Could you check a few things on this model? Use its own coordinates, in mm. A direction names the side the tool comes from. Give positions to 0.01 mm unless a question says otherwise; leave off trailing zeros. Loops run counter-clockwise (first coordinate to the right, second up) from the corner with the lowest first, then second, coordinate; pieces in that order, holes last. Notation, with made-up numbers: M 41.5,-28 L 99.5,-28 A29 cw 99.5,6 Z; hole C 68.25,7 d8. An arc over 180 degrees is marked long. Use a Markdown table: item, result. Add a question column.
1) Will this pin go through, and if not, where does the flat tip stop? pin 1 Ø2 at (x, z) = (3, -3) entering from +Y.
2) We'd pull the mould along X, two halves only. Please class faces 1 (the flat face through (6.35, 0, -6)), 2 (the flat face through (0.254, 3, -4)), 3 (the conical face through (4, 4, 11)), 4 (the conical face through (2.374, -0.513, -11.66)): +X half, -X half, draft (parallel to the pull), parting line (faces both ways), or undercut.
3) Suppose I cut it at C-C on x = 3.25. List the corners of the cut face in (y, z) for me (3 decimals).
4) If I drill on line 1 along Y through (x, z) = (0.1, 0) (1 decimal); line 2 along X through (y, z) = (-10.75, 9); line 3 along X through (y, z) = (-13, -6.75), over which ranges is the centre line in solid material (lowest first)? Write a range as [from, to].
5) Suppose I cut it at D-D on x = 1.5. List the corners of the cut face in (y, z) for me (3 decimals).
6) Which directions (+Z, -Z, +X, -X, +Y, -Y) give clear straight access to the entire face, cutting with the end or side of a thin tool? Please do faces 5 (the flat face through (6.096, -3, -4)), 6 (the cylindrical face through (3.22, 1.93, -2.52)).
```python
from build123d import *

# Parameters (mm, degrees)
SKETCH4_R          = 5.159375
SKETCH4_R_2        = 4.7625
CUT_EXTRUDE1_DEPTH = 0.254
CUT_EXTRUDE2_START = -0.254
SKETCH5_R          = 5.159375
SKETCH5_R_2        = 4.7625
CUT_EXTRUDE2_DEPTH = 0.254


with BuildPart() as part:
    # Sketch1 → Revolve1 (revolve)
    with BuildSketch(Plane.XY, mode=Mode.PRIVATE) as revolve1_sk:
        with BuildLine():
            Line((0, 3.175), (6.35, 3.175))
            Line((6.35, 3.175), (6.35, 14.816666667))
            ThreePointArc((6.35, 14.816666667), (6.279561395, 14.912197415), (6.167477521, 14.87314711))
            Line((6.167477521, 14.87314711), (3.830022177, 11.457936483))
            ThreePointArc((3.830022177, 11.457936483), (3.175, 11.1125), (2.519977823, 11.457936483))
            Line((2.519977823, 11.457936483), (0.182522479, 14.87314711))
            ThreePointArc((0.182522479, 14.87314711), (0.070438605, 14.912197415), (0, 14.816666667))
            Line((0, 14.816666667), (0, 3.175))
        make_face()
    revolve(revolve1_sk.sketch.rotate(Axis((0, 0, 0), (1, 0, 0)), 90), axis=Axis((0, 0, 0), (1, 0, 0)))

    # Sketch4 → Cut-Extrude1 (cut)
    with BuildSketch(Plane(origin=(6.35, 0, 0), x_dir=(0, 0, -1), z_dir=(1, 0, 0))):
        Circle(SKETCH4_R)
        Circle(SKETCH4_R_2, mode=Mode.SUBTRACT)
    extrude(amount=-CUT_EXTRUDE1_DEPTH, mode=Mode.SUBTRACT)

    # Sketch5 → Cut-Extrude2 (cut)
    with BuildSketch(Plane.ZY.offset(CUT_EXTRUDE2_START)):
        with Locations(Location((0, 0, 0), (0, 0, 180))):
            Circle(SKETCH5_R)
        with Locations(Location((0, 0, 0), (0, 0, 180))):
            Circle(SKETCH5_R_2, mode=Mode.SUBTRACT)
    extrude(amount=CUT_EXTRUDE2_DEPTH, mode=Mode.SUBTRACT)


solid = part.part
```
Answer block:
| question | item | result |
|---|---|---|
| 1 | pin 1 | stops at y = 11.86 |
| 2 | face 1 | +X half |
| 2 | face 2 | -X half |
| 2 | face 3 | undercut |
| 2 | face 4 | undercut |
| 3 | outline | C 0,0 d22.232; hole C 0,0 d6.35 |
| 4 | line 1 | y = [-14.9, -5.2], [-4.8, -3.2], [3.2, 4.8], [5.2, 14.9] |
| 4 | line 2 | x = [0, 0.77], [5.58, 6.35] |
| 4 | line 3 | x = [0, 0.34], [6.01, 6.35] |
| 5 | outline | C 0,0 d25.896; hole C 0,0 d6.35 |
| 6 | face 5 | +X |
| 6 | face 6 | +X, -X |
